```python
from build123d import *

# Parameters (mm, degrees)
SKETCH_1_W             = 51
SKETCH_1_H             = 25
SM_BASE_FLANGE_3_DEPTH = 2
OTHER_START            = -12.5
OTHER_3_DEPTH          = 25
OTHER_3_2_DEPTH        = 25
OTHER_4_DEPTH          = 25
OTHER_4_2_DEPTH        = 25
SKETCH_20_R            = 1.6
CUT_EXTRUDE_1_DEPTH    = 40
CUT_EXTRUDE_2_DEPTH    = 40
FILLET_1_R             = 3


# Read off the part's stored shape, not the designer's step: 绘制的折弯3, 绘制的折弯4
# Sheet-metal steps are written as plain solids
with BuildPart() as part:
    # 草图1 → 基体-法兰3 (new body)
    with BuildSketch(Plane(origin=(0, 0, 0), x_dir=(1, 0, 0), z_dir=(0, 1, 0))):
        Rectangle(SKETCH_1_W, SKETCH_1_H)
    extrude(amount=-SM_BASE_FLANGE_3_DEPTH)

    # Other 3 outline → Other 3 (cut)
    with BuildSketch(Plane.XY.offset(OTHER_START)):
        with BuildLine():
            Line((-25.5, -2), (-12.964101616, -2))
            ThreePointArc((-12.964101616, -2), (-11.5, -0.535898385), (-9.5, 0))
            Line((-9.5, 0), (-25.5, 0))
            Line((-25.5, 0), (-25.5, -2))
        make_face()
    extrude(amount=OTHER_3_DEPTH, mode=Mode.SUBTRACT)

    # Other 3 2 outline → Other 3 2 (add)
    with BuildSketch(Plane.XY.offset(OTHER_START)):
        with BuildLine():
            Line((-13.5, -15.28761102), (-11.5, -15.28761102))
            Line((-11.5, -15.28761102), (-11.5, -4))
            ThreePointArc((-11.5, -4), (-10.914213562, -2.585786438), (-9.5, -2))
            Line((-9.5, -2), (-12.964101616, -2))
            ThreePointArc((-12.964101616, -2), (-13.363703305, -2.96472382), (-13.5, -4))
            Line((-13.5, -4), (-13.5, -15.28761102))
        make_face()
    extrude(amount=OTHER_3_2_DEPTH)

    # Other 4 outline → Other 4 (cut)
    with BuildSketch(Plane.XY.offset(OTHER_START)):
        with BuildLine():
            ThreePointArc((9.5, 0), (11.5, -0.535898385), (12.964101616, -2))
            Line((12.964101616, -2), (25.5, -2))
            Line((25.5, -2), (25.5, 0))
            Line((25.5, 0), (9.5, 0))
        make_face()
    extrude(amount=OTHER_4_DEPTH, mode=Mode.SUBTRACT)

    # Other 4 2 outline → Other 4 2 (add)
    with BuildSketch(Plane.XY.offset(OTHER_START)):
        with BuildLine():
            Line((11.5, -4), (11.5, -15.28761102))
            Line((11.5, -15.28761102), (13.5, -15.28761102))
            Line((13.5, -15.28761102), (13.5, -4))
            ThreePointArc((13.5, -4), (13.363703305, -2.96472382), (12.964101616, -2))
            Line((12.964101616, -2), (9.5, -2))
            ThreePointArc((9.5, -2), (10.914213562, -2.585786438), (11.5, -4))
        make_face()
    extrude(amount=OTHER_4_2_DEPTH)

    # 草图20 → 切除-拉伸1 (cut)
    with BuildSketch(Plane(origin=(13.5, 0, 0), x_dir=(0, 0, -1), z_dir=(1, 0, 0))):
        with BuildLine():
            Line((-9.345, -9.64380551), (-7.745, -9.64380551))
            Line((-7.745, -9.64380551), (-6.145, -9.64380551))
            ThreePointArc((-6.145, -9.64380551), (-7.745, -8.04380551), (-9.345, -9.64380551))
        make_face()
        with BuildLine():
            Line((-6.145, -9.64380551), (-7.745, -9.64380551))
            Line((-7.745, -9.64380551), (-9.345, -9.64380551))
            ThreePointArc((-9.345, -9.64380551), (-7.745, -11.24380551), (-6.145, -9.64380551))
        make_face()
        with Locations(Location((7.745, -9.64380551, 0), (0, 0, 90))):
            Circle(SKETCH_20_R)
    extrude(amount=-CUT_EXTRUDE_1_DEPTH, mode=Mode.SUBTRACT)

    # 草图21 → 切除-拉伸2 (cut)
    with BuildSketch(Plane.XZ.offset(2)):
        with BuildLine():
            ThreePointArc((-5.25, 9.26), (-5.71862915, 10.39137085), (-6.85, 10.86))
            Line((-6.85, 10.86), (-6.85, 9.26))
            Line((-6.85, 9.26), (-5.25, 9.26))
        make_face()
        with BuildLine():
            Line((-5.25, 9.26), (-6.85, 9.26))
            Line((-6.85, 9.26), (-6.85, 7.66))
            ThreePointArc((-6.85, 7.66), (-5.71862915, 8.12862915), (-5.25, 9.26))
        make_face()
        with BuildLine():
            Line((-6.85, 9.26), (-6.85, 10.86))
            ThreePointArc((-6.85, 10.86), (-8.45, 9.26), (-6.85, 7.66))
            Line((-6.85, 7.66), (-6.85, 9.26))
        make_face()
        with BuildLine():
            Line((6.85, 9.26), (6.85, 10.86))
            ThreePointArc((6.85, 10.86), (5.71862915, 10.39137085), (5.25, 9.26))
            Line((5.25, 9.26), (6.85, 9.26))
        make_face()
        with BuildLine():
            Line((6.85, 7.66), (6.85, 9.26))
            Line((6.85, 9.26), (5.25, 9.26))
            ThreePointArc((5.25, 9.26), (5.71862915, 8.12862915), (6.85, 7.66))
        make_face()
        with BuildLine():
            ThreePointArc((8.45, 9.26), (7.98137085, 10.39137085), (6.85, 10.86))
            Line((6.85, 10.86), (6.85, 9.26))
            Line((6.85, 9.26), (6.85, 7.66))
            ThreePointArc((6.85, 7.66), (7.98137085, 8.12862915), (8.45, 9.26))
        make_face()
        with BuildLine():
            ThreePointArc((8.45, 0), (7.98137085, 1.13137085), (6.85, 1.6))
            Line((6.85, 1.6), (6.85, 0))
            Line((6.85, 0), (6.85, -1.6))
            ThreePointArc((6.85, -1.6), (7.98137085, -1.13137085), (8.45, 0))
        make_face()
        with BuildLine():
            Line((6.85, 0), (6.85, 1.6))
            ThreePointArc((6.85, 1.6), (5.25, 0), (6.85, -1.6))
            Line((6.85, -1.6), (6.85, 0))
        make_face()
        with BuildLine():
            ThreePointArc((-5.25, 0), (-5.71862915, 1.13137085), (-6.85, 1.6))
            Line((-6.85, 1.6), (-6.85, -1.6))
            ThreePointArc((-6.85, -1.6), (-5.71862915, -1.13137085), (-5.25, 0))
        make_face()
        with BuildLine():
            Line((-6.85, -1.6), (-6.85, 1.6))
            ThreePointArc((-6.85, 1.6), (-8.45, 0), (-6.85, -1.6))
        make_face()
        with BuildLine():
            ThreePointArc((-5.25, -9.26), (-5.71862915, -8.12862915), (-6.85, -7.66))
            Line((-6.85, -7.66), (-6.85, -9.26))
            Line((-6.85, -9.26), (-5.25, -9.26))
        make_face()
        with BuildLine():
            Line((-5.25, -9.26), (-6.85, -9.26))
            Line((-6.85, -9.26), (-6.85, -10.86))
            ThreePointArc((-6.85, -10.86), (-5.71862915, -10.39137085), (-5.25, -9.26))
        make_face()
        with BuildLine():
            Line((-6.85, -9.26), (-6.85, -7.66))
            ThreePointArc((-6.85, -7.66), (-8.45, -9.26), (-6.85, -10.86))
            Line((-6.85, -10.86), (-6.85, -9.26))
        make_face()
        with BuildLine():
            ThreePointArc((8.45, -9.26), (7.98137085, -8.12862915), (6.85, -7.66))
            Line((6.85, -7.66), (6.85, -9.26))
            Line((6.85, -9.26), (6.85, -10.86))
            ThreePointArc((6.85, -10.86), (7.98137085, -10.39137085), (8.45, -9.26))
        make_face()
        with BuildLine():
            Line((6.85, -9.26), (6.85, -7.66))
            ThreePointArc((6.85, -7.66), (5.71862915, -8.12862915), (5.25, -9.26))
            Line((5.25, -9.26), (6.85, -9.26))
        make_face()
        with BuildLine():
            Line((6.85, -10.86), (6.85, -9.26))
            Line((6.85, -9.26), (5.25, -9.26))
            ThreePointArc((5.25, -9.26), (5.71862915, -10.39137085), (6.85, -10.86))
        make_face()
    extrude(amount=-CUT_EXTRUDE_2_DEPTH, mode=Mode.SUBTRACT)

    # 圆角1
    fillet_1_edges = [part.edges().sort_by_distance(p)[0] for p in [
        (-12.5, -15.28761102, 12.5),
        (-12.5, -15.28761102, -12.5),
        (12.5, -15.28761102, -12.5),
        (12.5, -15.28761102, 12.5),
    ]]
    fillet(fillet_1_edges, radius=FILLET_1_R)


solid = part.part
```
Source: CAD feature listing. Evaluate the final solid. Frame: model axes, mm. A direction names the side the tool comes from. Give positions to 0.01 mm unless a question says otherwise; leave off trailing zeros. Loops run counter-clockwise (first coordinate to the right, second up) from the corner with the lowest first, then second, coordinate; pieces in that order, holes last. Notation, with made-up numbers: (76.5, -13) -> (80.5, -13) arc R28 cw to (80.5, 18) -> close; hole circle Ø9 at (3.5, -2). An arc over 180 degrees is marked (long way). Put each result on its own line as item: value. Start each with the question number.
1) Draft query along Z for faces 3 (the face through (-11.5, -10, 0)), 4 (the face through (0, -1, -12.5)), 5 (the face through (12.514, -11.242, -7.675)). Return one class per face: released by +Z, released by -Z, zero draft, split by the parting line, or undercut.
2) Cut plane D-D (x = -4.75). Return loops of the section in (y, z).
3) Cut plane C-C (z = 10). Return loops of the section in (x, y).
4) Reachability of faces 1 (the face through (-10.93, -2.6, -0.18)), 2 (the face through (12, -15.288, 0)) from +Z, -Z, +X, -X, +Y, -Y: full face, straight path, thin tool, end or side. Return the list, or none.
5) Cut plane A-A (y = -7.5). Return loops of the section in (x, z), then the cut area to 3 significant figures.
6) Material intervals for probe 1 along X at (y, z) = (-8, 11); probe 2 along Z at (x, y) = (8, -0.5); probe 3 along Y at (x, z) = (3, 5), sorted ascending.
7) Contact query for a flat-ended pin moving along its axis: P1, Ø4, axis at x = 2.5, z = 8, coming from the -Y side. Output: stop coordinate, or through.
8) Cut plane B-B (z = -6.5). Return loops of the section in (x, y).
Results are:
1. face 3: zero draft
1. face 4: released by -Z
1. face 5: undercut
2. outline: (-2, -12.5) -> (0, -12.5) -> (0, 12.5) -> (-2, 12.5) -> close
3. outline: (-13.5, -15.25) -> (-11.5, -15.25) -> (-11.5, -4) arc R2 cw to (-9.5, -2) -> (-8.27, -2) -> (-8.27, 0) -> (-9.5, 0) arc R4 ccw to (-13.5, -4) -> close; (-5.43, -2) -> (5.43, -2) -> (5.43, 0) -> (-5.43, 0) -> close; (8.27, -2) -> (9.5, -2) arc R2 cw to (11.5, -4) -> (11.5, -15.25) -> (13.5, -15.25) -> (13.5, -4) arc R4 ccw to (9.5, 0) -> (8.27, 0) -> close
4. face 1: +Z, -Z, -Y
4. face 2: +Z, -Z, +X, -X, -Y
5. outline: (-13.5, -12.5) -> (-11.5, -12.5) -> (-11.5, 12.5) -> (-13.5, 12.5) -> close; (11.5, -12.5) -> (13.5, -12.5) -> (13.5, 12.5) -> (11.5, 12.5) -> close
5. area: 100 mm2
6. probe 1: x = -13.5 to -11.5, 11.5 to 13.5
6. probe 2: z = -12.5 to -10.37, -8.15 to -1.11, 1.11 to 8.15, 10.37 to 12.5
6. probe 3: y = -2 to 0
7. P1: stops at y = -2
8. outline: (-13.5, -15.29) -> (-11.5, -15.29) -> (-11.5, -10.65) -> (-13.5, -10.65) -> close; (-13.5, -8.64) -> (-11.5, -8.64) -> (-11.5, -4) arc R2 cw to (-9.5, -2) -> (9.5, -2) arc R2 cw to (11.5, -4) -> (11.5, -8.64) -> (13.5, -8.64) -> (13.5, -4) arc R4 ccw to (9.5, 0) -> (-9.5, 0) arc R4 ccw to (-13.5, -4) -> close; (11.5, -15.29) -> (13.5, -15.29) -> (13.5, -10.65) -> (11.5, -10.65) -> close
